Answer from the drawing. Dimensions are ordinates in mm from the lowest x, y and z of the part. A direction names the side the tool comes from. Round coordinates to 2 decimals unless told otherwise and drop trailing zeros. Order: outer loops, then holes, each group sorted by start corner. A loop starts at its lowest first (then second) coordinate and runs counter-clockwise, first axis right, second up. Notation, with made-up numbers: (89.5, 83) -> (103.5, 83) arc R12 cw to (103.5, 101) -> close; hole circle Ø1 at (33.25, 24). An arc over 180 degrees is marked (long way). Use a Markdown table: item, result. Add a question column.
1. The mould has two halves that part along X. Classify the marked faces 4, 5 and 6: +X half, -X half, draft (parallel to the pull), parting line (faces both ways), or undercut.
2. Given pin 1 (1 mm diameter, centred on x = 6, z = 14, fed in from -Y); pin 2 (2 mm diameter, centred on x = 5.5, y = 16.5, fed in from -Z); pin 3 (10 mm diameter, centred on x = 14.5, z = 6.5, fed in from +Y); pin 4 (1.5 mm diameter, centred on x = 4.5, y = 9.5, fed in from +Z), each flat-ended and moving along its own axis, determine where each tip first touches the part or whether it passes through.
3. Section D-D, the plane y = 21 is taken. Give the vertices of the cut face in (x, z).
4. Section A-A, the plane x = 10.5 is taken. Give the vertices of the cut face in (y, z), then the cut area to 3 significant figures.
5. Consider L1, parallel to Y at x = 17.5, z = 30; L2, parallel to Y at x = 18, z = 14 (1 decimal); L3, parallel to Z at x = 10, y = 26 (1 decimal). Determine where each line is inside the solid, lowest interval first. Write a range as [from, to].
6. For the marked faces 1, 2 and 3, determine the directions among +Z, -Z, +X, -X, +Y, -Y from which every point of the face is accessible in a straight line to the end or side of a thin tool.
7. Section C-C, the plane x = 7 is taken. Give the vertices of the cut face in (y, z).
8. Section B-B, the plane z = 19 is taken. Give the vertices of the cut face in (x, y), then the cut area to 3 significant figures.
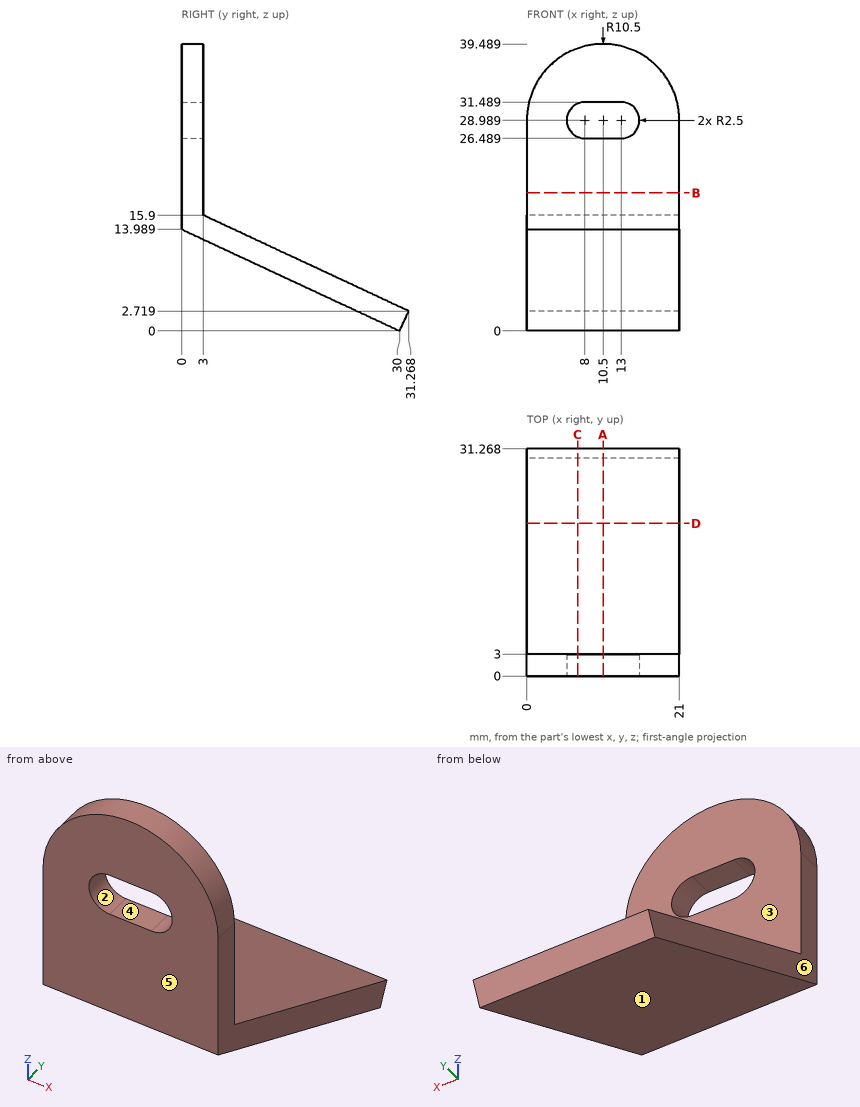
Verdict:
| question | item | result |
|---|---|---|
| 1 | face 4 | undercut |
| 1 | face 5 | draft |
| 1 | face 6 | -X half |
| 2 | pin 1 | stops at y = 0 |
| 2 | pin 2 | stops at z = 5.83 |
| 2 | pin 3 | stops at y = 31.27 |
| 2 | pin 4 | stops at z = 13.22 |
| 3 | outline | (0, 4.2) -> (21, 4.2) -> (21, 7.51) -> (0, 7.51) -> close |
| 4 | outline | (0, 13.99) -> (30, 0) -> (31.27, 2.72) -> (3, 15.9) -> (3, 26.49) -> (0, 26.49) -> close; (0, 31.49) -> (3, 31.49) -> (3, 39.49) -> (0, 39.49) -> close |
| 4 | area | 155 mm2 |
| 5 | L1 | y = [0, 3] |
| 5 | L2 | y = [0, 7.1] |
| 5 | L3 | z = [1.9, 5.2] |
| 6 | face 1 | -Z, +X, -X, -Y |
| 6 | face 2 | +Y, -Y |
| 6 | face 3 | +Z, +X, -X, +Y |
| 7 | outline | (0, 13.99) -> (30, 0) -> (31.27, 2.72) -> (3, 15.9) -> (3, 26.7) -> (0, 26.7) -> close; (0, 31.28) -> (3, 31.28) -> (3, 38.89) -> (0, 38.89) -> close |
| 8 | outline | (0, 0) -> (21, 0) -> (21, 3) -> (0, 3) -> close |
| 8 | area | 63.0 mm2 |
